```python
from build123d import *

# Parameters (mm, degrees)
SKETCH_1_W          = 550
SKETCH_1_H          = 300
SKETCH_1_W_2        = 350
SKETCH_1_H_2        = 40
EXTRUDE_1_DEPTH     = 20
CHAMFER_1_SIZE      = 5
SKETCH_2_R          = 5
CUT_EXTRUDE_1_DEPTH = 17


with BuildPart() as part:
    # Эскиз1 → Бобышка-Вытянуть1 (new body)
    with BuildSketch(Plane(origin=(0, 0, 0), x_dir=(1, 0, 0), z_dir=(0, 1, 0))):
        Rectangle(SKETCH_1_W, SKETCH_1_H)
        Rectangle(SKETCH_1_W_2, SKETCH_1_H_2, mode=Mode.SUBTRACT)
    extrude(amount=-EXTRUDE_1_DEPTH)

    # Фаска1
    chamfer_1_edges = [part.edges().sort_by_distance(p)[0] for p in [
        (275, -10, 150),
        (-275, -10, 150),
        (-275, -10, -150),
        (275, -10, -150),
    ]]
    chamfer(chamfer_1_edges, length=CHAMFER_1_SIZE)

    # Эскиз2 → Вырез-Вытянуть1 (cut)
    with BuildSketch(Plane(origin=(0, -20, 0), x_dir=(-1, 0, 0), z_dir=(0, 1, 0))):
        with Locations(Location((240, 115, 0), (0, 0, 270))):
            Circle(SKETCH_2_R)
        with Locations(Location((-240, 115, 0), (0, 0, 270))):
            Circle(SKETCH_2_R)
        with Locations(Location((-240, -115, 0), (0, 0, 270))):
            Circle(SKETCH_2_R)
        with Locations(Location((240, -115, 0), (0, 0, 270))):
            Circle(SKETCH_2_R)
    extrude(amount=CUT_EXTRUDE_1_DEPTH, mode=Mode.SUBTRACT)


solid = part.part
```
Verification items for the finished model (mm, model axes). A direction names the side the tool comes from. Coordinates: 2 decimals unless noted, no trailing zeros. Write each loop counter-clockwise with the first axis right and the second up, starting at its lowest first coordinate (ties: lowest second). Pieces come first, ordered by that corner, then holes. Notation, with made-up numbers: M 20.5,16.25 L 68.5,16.25 A22 cw 68.5,39.25 Z; hole C 27.25,8 d11. An arc over 180 degrees is marked long. One line per item, written item: value.
Item 1: Scan lines: line 1 along X through (y, z) = (-12.75, -115); line 2 along Z through (x, y) = (-240, -14); line 3 along X through (y, z) = (-5, 116). Record each from-to range of solid material in increasing order.
Check sheet entries:
line 1: x = -275 to -245, -235 to 235, 245 to 275
line 2: z = -150 to -120, -110 to 110, 120 to 150
line 3: x = -275 to -244.9, -235.1 to 235.1, 244.9 to 275
Item 2: Section check C-C, the plane y = -13.5. Record the boundary of the cut face in (x, z).
Check sheet entries:
outline: M -275,-145 L -270,-150 L 270,-150 L 275,-145 L 275,145 L 270,150 L -270,150 L -275,145 Z; hole C -240,-115 d10; hole C -240,115 d10; hole M -175,-20 L 175,-20 L 175,20 L -175,20 Z; hole C 240,-115 d10; hole C 240,115 d10
Item 3: Section check A-A, the plane z = 8. Record the boundary of the cut face in (x, y), plus the area to 3 significant figures.
Check sheet entries:
outline: M -275,-20 L -175,-20 L -175,0 L -275,0 Z; M 175,-20 L 275,-20 L 275,0 L 175,0 Z
area: 4,000 mm^2
Item 4: Section check B-B, the plane x = -38. Record the boundary of the cut face in (y, z), plus the area to 3 significant figures.
Check sheet entries:
outline: M -20,-150 L 0,-150 L 0,-20 L -20,-20 Z; M -20,20 L 0,20 L 0,150 L -20,150 Z
area: 5,200 mm^2
Item 5: Gauge pin test, flat ends, axial feed: pin 1 Ø16 at (x, z) = (240, -115) entering from +Y; pin 2 Ø6 at (x, z) = (-240, -115) entering from -Y. Record the tip position at first contact, or that the pin passes through.
Check sheet entries:
pin 1: stops at y = 0
pin 2: stops at y = -3
Item 6: Access from +Z, -Z, +X, -X, +Y, -Y to the whole of each face (thin tool, end or side, straight path). Record for faces 1 (the flat face through (175, -10, 0)), 2 (the flat face through (-240, -3, 115)), 3 (the flat face through (-275, -10, 2)).
Check sheet entries:
face 1: +Y, -Y
face 2: -Y
face 3: +Z, -Z, -X, +Y, -Y
